Geometry: final body of the model. Coordinates: model frame, mm. A direction names the side the tool comes from. Give positions to 0.01 mm unless a question says otherwise; leave off trailing zeros.
Q1. Draft query along Y for faces 5 (the face through (-8, -12.7, 213)), 6 (the face through (-4.572, 0, 213)), 7 (the face through (-12.7, 8, 213)). Return one class per face: pulls with the +Y half, pulls with the -Y half, needs draft (parallel to the pull), parting line crosses it, or undercut.
Q2. Line query: L1, parallel to Y at x = 7.75, z = 74; L2, parallel to Y at x = 0, z = 100. Output: solid intervals per line, ascending.
Q3. Pin query (flat end, axial travel): pin 1 (1 mm diameter, centred on x = -0.5, z = 114.5, fed in from +Y); pin 2 (1 mm diameter, centred on x = 5.5, y = -1, fed in from -Z). Return the tip coordinate at first contact, or that it passes through.
Q4. Reachability of faces 1 (the face through (4.572, 0, 213)), 2 (the face through (0, -4.572, 213)), 3 (the face through (8, -12.7, 213)), 4 (the face through (0, 4.572, 213)) from +Z, -Z, +X, -X, +Y, -Y: full face, straight path, thin tool, end or side. Return the list, or none.
```python
from build123d import *

# Parameters (mm, degrees)
F0_R     = 2.794
F1_DEPTH = 431.8


with BuildPart() as f1:
    # F0 (on Top) → F1 (new body)
    with BuildSketch(Plane.XY):
        Polygon((4.572, -3.440488), (4.572, -4.572), (3.440488, -4.572), (6.604, -7.735512), (6.604, -10.414), (10.414, -10.414), (10.414, -6.604), (7.735512, -6.604), align=None)
        Polygon((3.440488, -4.572), (4.572, -4.572), (4.572, -3.440488), (4.572, 3.440488), (4.572, 4.572), (3.440488, 4.572), (-3.440488, 4.572), (-4.572, 4.572), (-4.572, 3.440488), (-4.572, -3.440488), (-4.572, -4.572), (-3.440488, -4.572), align=None)
        Circle(F0_R, mode=Mode.SUBTRACT)
        Polygon((-6.604, -7.735512), (-3.440488, -4.572), (-4.572, -4.572), (-4.572, -3.440488), (-7.735512, -6.604), (-10.414, -6.604), (-10.414, -10.414), (-6.604, -10.414), align=None)
        Polygon((4.572, 4.572), (4.572, 3.440488), (7.735512, 6.604), (10.414, 6.604), (10.414, 10.414), (6.604, 10.414), (6.604, 7.735512), (3.440488, 4.572), align=None)
        with BuildLine():
            Line((10.414, -10.414), (6.604, -10.414))
            Line((6.604, -10.414), (4.92125, -10.414))
            ThreePointArc((4.92125, -10.414), (4.064, -11.557), (4.92125, -12.7))
            Line((4.92125, -12.7), (10.414, -12.7))
            Line((10.414, -12.7), (10.414, -10.414))
        make_face()
        with BuildLine():
            Line((10.414, -4.92125), (10.414, -6.604))
            Line((10.414, -6.604), (10.414, -10.414))
            Line((10.414, -10.414), (12.7, -10.414))
            Line((12.7, -10.414), (12.7, -4.92125))
            ThreePointArc((12.7, -4.92125), (11.557, -4.064), (10.414, -4.92125))
        make_face()
        with BuildLine():
            Line((-4.92125, -10.414), (-6.604, -10.414))
            Line((-6.604, -10.414), (-10.414, -10.414))
            Line((-10.414, -10.414), (-10.414, -12.7))
            Line((-10.414, -12.7), (-4.92125, -12.7))
            ThreePointArc((-4.92125, -12.7), (-4.064, -11.557), (-4.92125, -10.414))
        make_face()
        with BuildLine():
            Line((12.7, -10.414), (10.414, -10.414))
            Line((10.414, -10.414), (10.414, -12.7))
            Line((10.414, -12.7), (11.43, -12.7))
            ThreePointArc((11.43, -12.7), (12.328026, -12.328026), (12.7, -11.43))
            Line((12.7, -11.43), (12.7, -10.414))
        make_face()
        with BuildLine():
            Line((10.414, 10.414), (10.414, 6.604))
            Line((10.414, 6.604), (10.414, 4.92125))
            ThreePointArc((10.414, 4.92125), (11.557, 4.064), (12.7, 4.92125))
            Line((12.7, 4.92125), (12.7, 10.414))
            Line((12.7, 10.414), (10.414, 10.414))
        make_face()
        Polygon((-7.735512, 6.604), (-4.572, 3.440488), (-4.572, 4.572), (-3.440488, 4.572), (-6.604, 7.735512), (-6.604, 10.414), (-10.414, 10.414), (-10.414, 6.604), align=None)
        with BuildLine():
            Line((-12.7, -10.414), (-10.414, -10.414))
            Line((-10.414, -10.414), (-10.414, -6.604))
            Line((-10.414, -6.604), (-10.414, -4.92125))
            ThreePointArc((-10.414, -4.92125), (-11.557, -4.064), (-12.7, -4.92125))
            Line((-12.7, -4.92125), (-12.7, -10.414))
        make_face()
        with BuildLine():
            Line((-10.414, -12.7), (-10.414, -10.414))
            Line((-10.414, -10.414), (-12.7, -10.414))
            Line((-12.7, -10.414), (-12.7, -11.43))
            ThreePointArc((-12.7, -11.43), (-12.328026, -12.328026), (-11.43, -12.7))
            Line((-11.43, -12.7), (-10.414, -12.7))
        make_face()
        with BuildLine():
            Line((10.414, 12.7), (10.414, 10.414))
            Line((10.414, 10.414), (12.7, 10.414))
            Line((12.7, 10.414), (12.7, 11.43))
            ThreePointArc((12.7, 11.43), (12.328026, 12.328026), (11.43, 12.7))
            Line((11.43, 12.7), (10.414, 12.7))
        make_face()
        with BuildLine():
            Line((6.604, 10.414), (10.414, 10.414))
            Line((10.414, 10.414), (10.414, 12.7))
            Line((10.414, 12.7), (4.92125, 12.7))
            ThreePointArc((4.92125, 12.7), (4.064, 11.557), (4.92125, 10.414))
            Line((4.92125, 10.414), (6.604, 10.414))
        make_face()
        with BuildLine():
            Line((-10.414, 4.92125), (-10.414, 6.604))
            Line((-10.414, 6.604), (-10.414, 10.414))
            Line((-10.414, 10.414), (-12.7, 10.414))
            Line((-12.7, 10.414), (-12.7, 4.92125))
            ThreePointArc((-12.7, 4.92125), (-11.557, 4.064), (-10.414, 4.92125))
        make_face()
        with BuildLine():
            Line((-10.414, 10.414), (-6.604, 10.414))
            Line((-6.604, 10.414), (-4.92125, 10.414))
            ThreePointArc((-4.92125, 10.414), (-4.064, 11.557), (-4.92125, 12.7))
            Line((-4.92125, 12.7), (-10.414, 12.7))
            Line((-10.414, 12.7), (-10.414, 10.414))
        make_face()
        with BuildLine():
            Line((-12.7, 10.414), (-10.414, 10.414))
            Line((-10.414, 10.414), (-10.414, 12.7))
            Line((-10.414, 12.7), (-11.43, 12.7))
            ThreePointArc((-11.43, 12.7), (-12.328026, 12.328026), (-12.7, 11.43))
            Line((-12.7, 11.43), (-12.7, 10.414))
        make_face()
    extrude(amount=F1_DEPTH)


solid = f1.part
```
Data:
1. face 5: pulls with the -Y half
1. face 6: undercut
1. face 7: needs draft
2. L1: y = -12.7 to -6.6, 6.6 to 12.7
2. L2: y = -4.57 to -2.79, 2.79 to 4.57
3. pin 1: stops at y = 4.57
3. pin 2: passes through
4. face 1: +Z, -Z, +X
4. face 2: +Z, -Z, -Y
4. face 3: +Z, -Z, +X, -X, -Y
4. face 4: +Z, -Z, +Y
